For this review, take the finished solid that the model builds, in its own axes (mm). Face numbers are marked on the shaded views. Coordinates: 2 decimals unless noted, no trailing zeros. Write each loop counter-clockwise with the first axis right and the second up, starting at its lowest first coordinate (ties: lowest second). Pieces come first, ordered by that corner, then holes. Notation, with made-up numbers: (62, 42) -> (72, 42) arc R25 cw to (72, 66) -> close; hole circle Ø8 at (36.5, -11.75). An arc over 180 degrees is marked (long way). One line per item, written item: value. Start each with the question number.
1) Mouldability with a two-part tool opening along Y and no side actions: class the marked faces 1 and 2 as released by +Y, released by -Y, zero draft, split by the parting line, or undercut.
2) Add section B-B (x = 19.05). State the section outline as (y, z) points (3 decimals).
3) For probe 1 along Y at (x, z) = (19.05, 0.85) (3 decimals); probe 2 along Z at (x, y) = (25.5, -15); probe 3 along Y at (x, z) = (-7, 7.5), list the stretches that pass through material, from the lowest coordinate up. Write a range as from..to.
4) Add section D-D (x = 2). State the section outline as (y, z) points.
5) For pin 1 Ø8 at (x, y) = (-4.5, -1.5) entering from -Z; pin 2 Ø10 at (x, y) = (21, 8) entering from +Z; pin 3 Ø2.5 at (x, z) = (-6, 7.5) entering from -Y, all flat-tipped, find the tip position at first contact; note any pin that passes through.
6) Add section C-C (y = -4.5). State the section outline as (x, z) points.
7) Add section A-A (y = 0). State the section outline as (x, z) points (3 decimals), and give its area (3 significant figures).
from build123d import *

# Parameters (mm, degrees)
F0_W     = 53.467
F0_H     = 35.814
F0_R     = 1.905
F1_DEPTH = 1.6002
F2_W     = 25.4
F2_H     = 10.16
F3_DEPTH = 8.128


with BuildPart() as f1:
    # F0 (on Top) → F1 (new body)
    with BuildSketch(Plane.XY):
        with Locations((2.6035, 1.397)):
            Rectangle(F0_W, F0_H)
        with Locations((-19.05, 0)):
            Circle(F0_R, mode=Mode.SUBTRACT)
        with Locations((19.05, 0)):
            Circle(F0_R, mode=Mode.SUBTRACT)
    extrude(amount=F1_DEPTH)

    # F2 (on face) → F3 (join)
    with BuildSketch(Plane.XY.offset(1.6002)):
        Rectangle(F2_W, F2_H)
    extrude(amount=F3_DEPTH)


solid = f1.part
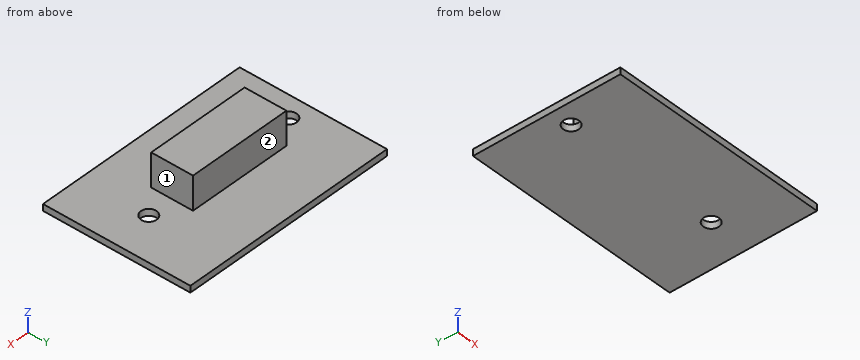
Numbers:
1. face 1: zero draft
1. face 2: released by +Y
2. outline: (-16.51, 0) -> (-1.905, 0) -> (-1.905, 1.6) -> (-16.51, 1.6) -> close; (1.905, 0) -> (19.304, 0) -> (19.304, 1.6) -> (1.905, 1.6) -> close
3. probe 1: -16.51..-1.905, 1.905..19.304
3. probe 2: 0..1.6
3. probe 3: -5.08..5.08
4. outline: (-16.51, 0) -> (19.3, 0) -> (19.3, 1.6) -> (5.08, 1.6) -> (5.08, 9.73) -> (-5.08, 9.73) -> (-5.08, 1.6) -> (-16.51, 1.6) -> close
5. pin 1: z = 0
5. pin 2: z = 1.6
5. pin 3: y = -5.08
6. outline: (-24.13, 0) -> (29.34, 0) -> (29.34, 1.6) -> (12.7, 1.6) -> (12.7, 9.73) -> (-12.7, 9.73) -> (-12.7, 1.6) -> (-24.13, 1.6) -> close
7. outline: (-24.13, 0) -> (-20.955, 0) -> (-20.955, 1.6) -> (-24.13, 1.6) -> close; (-17.145, 0) -> (17.145, 0) -> (17.145, 1.6) -> (12.7, 1.6) -> (12.7, 9.728) -> (-12.7, 9.728) -> (-12.7, 1.6) -> (-17.145, 1.6) -> close; (20.955, 0) -> (29.337, 0) -> (29.337, 1.6) -> (20.955, 1.6) -> close
7. area: 280 mm²
